Can you work these out from the drawing? Everything is in mm from the part's minimum corner. A direction names the side the tool comes from. Coordinates: 2 decimals unless noted, no trailing zeros. Order: outer loops, then holes, each group sorted by start corner. A loop starts at its lowest first (then second) coordinate and runs counter-clockwise, first axis right, second up. Notation, with made-up numbers: (25, -19.5) -> (37, -19.5) arc R18 ccw to (37, 15.5) -> close; hole circle Ø5 at (-27, 34). An arc over 180 degrees is marked (long way). Use a Markdown table: item, result. Add a question column.
1) Which directions (+Z, -Z, +X, -X, +Y, -Y) give clear straight access to the entire face, cutting with the end or side of a thin tool? Please do the marked faces 1, 2 and 3.
2) If we section it at C-C (x = 3.6): Write out the boundary of the cut face in (y, z).
3) If we section it at A-A (y = 10.25): Write out the boundary of the cut face in (x, z), plus the area to 3 significant figures.
4) If we section it at B-B (z = 5.35): Write out the boundary of the cut face in (x, y), plus the area to 3 significant figures.
5) Will this pin go through, and if not, where does the flat tip stop? pin 1 Ø1 at (x, y) = (5, 16.5) entering from +Z.
6) If I drill on L1, parallel to Y at x = 5.4, z = 5.55; L2, parallel to Y at x = 4.45, z = 2.4; L3, parallel to Z at x = 4.45, y = 1, over which ranges is the centre line in solid material (lowest first)? Write a range as [from, to].
7) If we section it at D-D (z = 1.3): Write out the boundary of the cut face in (x, y).
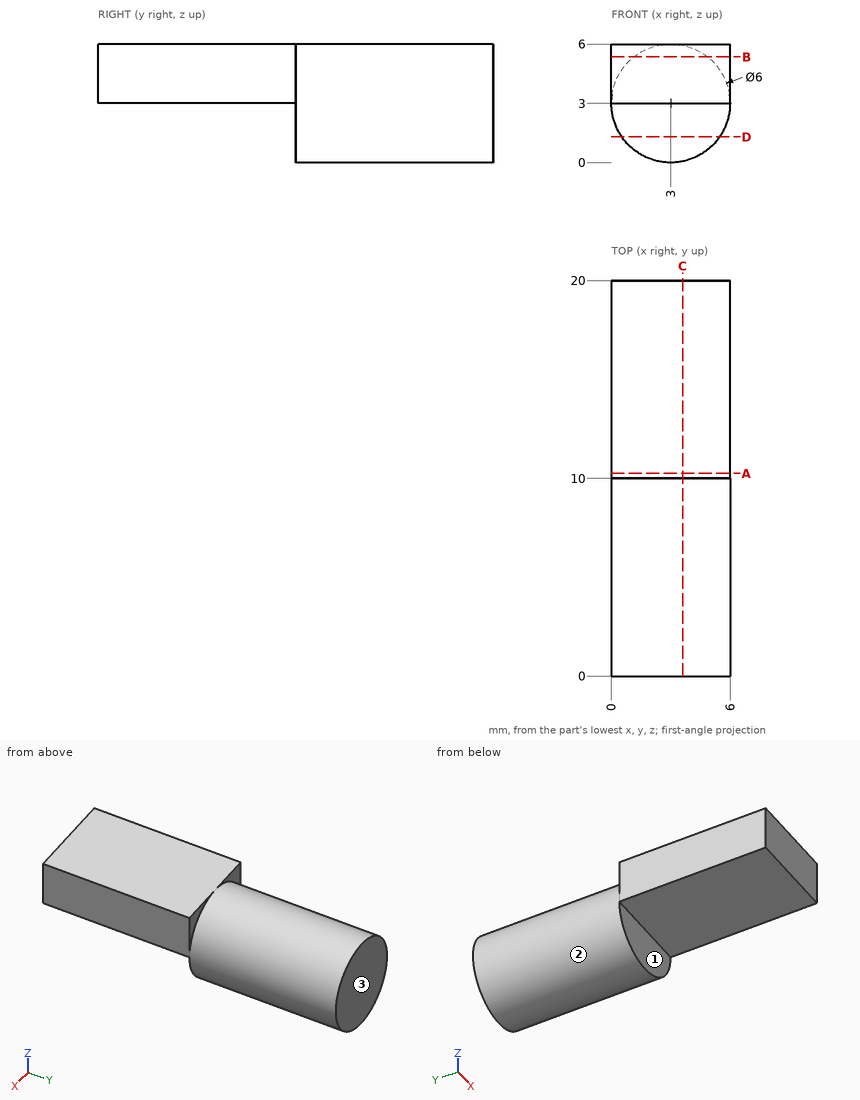
Answer sheet:
| question | item | result |
|---|---|---|
| 1 | face 1 | -Z, +X, -X, -Y |
| 1 | face 2 | +Y |
| 1 | face 3 | +Z, -Z, +X, -X, +Y |
| 2 | outline | (0, 3) -> (10, 3) -> (10, 0.06) -> (20, 0.06) -> (20, 5.94) -> (10, 5.94) -> (10, 6) -> (0, 6) -> close |
| 3 | outline | circle Ø6 at (3, 3) |
| 3 | area | 28.3 mm2 |
| 4 | outline | (0, 0) -> (6, 0) -> (6, 10) -> (4.86, 10) -> (4.86, 20) -> (1.14, 20) -> (1.14, 10) -> (0, 10) -> close |
| 4 | area | 97.3 mm2 |
| 5 | pin 1 | z = 5.6 |
| 6 | L1 | [0, 10] |
| 6 | L2 | [10, 20] |
| 6 | L3 | [3, 6] |
| 7 | outline | (0.53, 10) -> (5.47, 10) -> (5.47, 20) -> (0.53, 20) -> close |
